```python
from build123d import *

# Parameters (mm, degrees)
SKETCH1_W           = 199
SKETCH1_H           = 129.3
SKETCH1_R           = 7.9
SKETCH1_R_2         = 3.5
SKETCH1_W_2         = 2.25
SKETCH1_H_2         = 2.25
BOSS_EXTRUDE1_DEPTH = 2.13


with BuildPart() as part:
    # Sketch1 → Boss-Extrude1 (new body)
    with BuildSketch(Plane(origin=(0, 0, 0), x_dir=(1, 0, 0), z_dir=(0, 1, 0))):
        Rectangle(SKETCH1_W, SKETCH1_H)
        with Locations((-70, 45)):
            Circle(SKETCH1_R, mode=Mode.SUBTRACT)
        with Locations((-35, 45)):
            Circle(SKETCH1_R, mode=Mode.SUBTRACT)
        with Locations((0, 45)):
            Circle(SKETCH1_R, mode=Mode.SUBTRACT)
        with Locations((35, 45)):
            Circle(SKETCH1_R, mode=Mode.SUBTRACT)
        with Locations((-35, 15)):
            Circle(SKETCH1_R, mode=Mode.SUBTRACT)
        with Locations((0, 15)):
            Circle(SKETCH1_R, mode=Mode.SUBTRACT)
        with Locations((35, 15)):
            Circle(SKETCH1_R, mode=Mode.SUBTRACT)
        with Locations((-35, -15)):
            Circle(SKETCH1_R, mode=Mode.SUBTRACT)
        with Locations((0, -15)):
            Circle(SKETCH1_R, mode=Mode.SUBTRACT)
        with Locations((35, -15)):
            Circle(SKETCH1_R, mode=Mode.SUBTRACT)
        with Locations((-35, -45)):
            Circle(SKETCH1_R, mode=Mode.SUBTRACT)
        with Locations((0, -45)):
            Circle(SKETCH1_R, mode=Mode.SUBTRACT)
        with Locations((35, -45)):
            Circle(SKETCH1_R, mode=Mode.SUBTRACT)
        with Locations((-70, 15)):
            Circle(SKETCH1_R, mode=Mode.SUBTRACT)
        with Locations((-70, -15)):
            Circle(SKETCH1_R, mode=Mode.SUBTRACT)
        with Locations((-70, -45)):
            Circle(SKETCH1_R, mode=Mode.SUBTRACT)
        with Locations((70, 35)):
            Circle(SKETCH1_R_2, mode=Mode.SUBTRACT)
        with Locations((70, 0)):
            Circle(SKETCH1_R_2, mode=Mode.SUBTRACT)
        with Locations((70, -35)):
            Circle(SKETCH1_R_2, mode=Mode.SUBTRACT)
        with Locations((70, 43.125)):
            Rectangle(SKETCH1_W_2, SKETCH1_H_2, mode=Mode.SUBTRACT)
        with Locations((70, 8.125)):
            Rectangle(SKETCH1_W_2, SKETCH1_H_2, mode=Mode.SUBTRACT)
        with Locations((70, -26.875)):
            Rectangle(SKETCH1_W_2, SKETCH1_H_2, mode=Mode.SUBTRACT)
    extrude(amount=BOSS_EXTRUDE1_DEPTH)


solid = part.part
```
Build history of the part. All positions in model axes, mm. Coordinates: 2 decimals unless noted, no trailing zeros. Write each loop counter-clockwise with the first axis right and the second up, starting at its lowest first coordinate (ties: lowest second). Pieces come first, ordered by that corner, then holes.
1. Band-saw the part on B-B, the plane x = -35. Give the cut face in (y, z), and give its area (3 significant figures).
Answer block:
outline: (0, -64.65) - (2.13, -64.65) - (2.13, -52.9) - (0, -52.9) - close; (0, -37.1) - (2.13, -37.1) - (2.13, -22.9) - (0, -22.9) - close; (0, -7.1) - (2.13, -7.1) - (2.13, 7.1) - (0, 7.1) - close; (0, 22.9) - (2.13, 22.9) - (2.13, 37.1) - (0, 37.1) - close; (0, 52.9) - (2.13, 52.9) - (2.13, 64.65) - (0, 64.65) - close
area: 141 mm2
2. Pull direction Z, two halves, no side cores. Call faces 1 (the cylindrical face through (67.42, 1.05, -37.365)), 2 (the flat face through (-1, 0, -1)): released by +Z, released by -Z, zero draft, split by the parting line, or undercut.
Answer block:
face 1: undercut
face 2: zero draft
3. Drill centre lines: probe 1 along Z at (x, y) = (35, 0.6); probe 2 along X at (y, z) = (0.7, 45); probe 3 along X at (y, z) = (0.5, 19). Where is each one in solid material? Low to high.
Answer block:
probe 1: z = -64.65 to -52.9, -37.1 to -22.9, -7.1 to 7.1, 22.9 to 37.1, 52.9 to 64.65
probe 2: x = -99.5 to -77.9, -62.1 to -42.9, -27.1 to -7.9, 7.9 to 27.1, 42.9 to 99.5
probe 3: x = -99.5 to -76.81, -63.19 to -41.81, -28.19 to -6.81, 6.81 to 28.19, 41.81 to 99.5
4. Band-saw the part on C-C, the plane y = 0.35. Give the number of separate pieces and of enclosed holes in the cut face, and give its area (3 significant figures).
Answer block:
separate pieces: 1
enclosed holes: 22
area: 22,500 mm2
5. Band-saw the part on A-A, the plane z = -35. Give the cut face in (x, y).
Answer block:
outline: (-99.5, 0) - (66.5, 0) - (66.5, 2.13) - (-99.5, 2.13) - close; (73.5, 0) - (99.5, 0) - (99.5, 2.13) - (73.5, 2.13) - close
